Here's the drawing with two shaded views (mm, measured from the low corner). I have some questions. Round coordinates to 2 decimals unless told otherwise and drop trailing zeros.
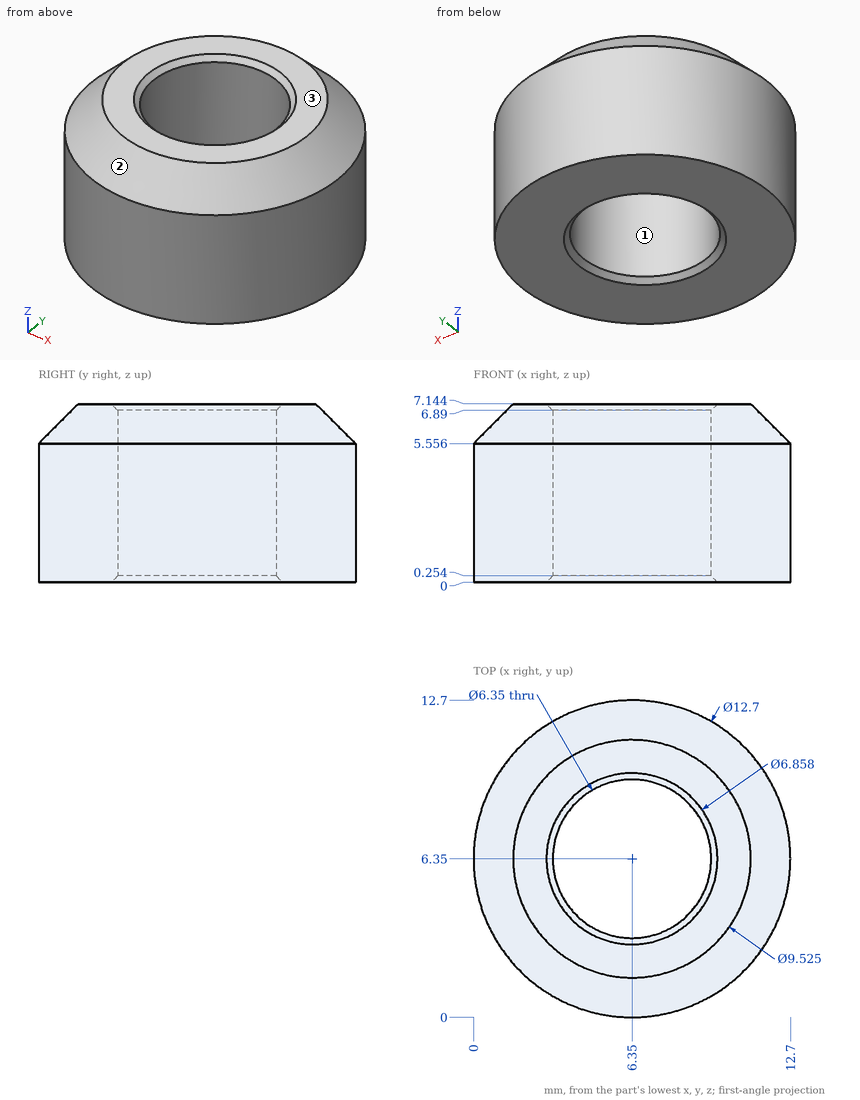
Item 1: Will these pins go through, and if not, where does the flat tip stop? pin 1 (5.5 mm diameter, centred on x = 6.35, y = 6.35, fed in from -Z); pin 2 (3 mm diameter, centred on x = 4, z = 6.5, fed in from -Y); pin 3 (2 mm diameter, centred on x = 3.5, z = 4, fed in from -Y) (1 decimal); pin 4 (2 mm diameter, centred on x = 10.5, z = 3, fed in from -Y).
Results list:
pin 1: passes through
pin 2: stops at y = 0.11
pin 3: stops at y = 0.3
pin 4: stops at y = 0.84
Item 2: If I drill on line 1 along Y through (x, z) = (6.35, 3.5) (1 decimal); line 2 along Y through (x, z) = (7.75, 0.75); line 3 along X through (y, z) = (8.75, 2.75), over which ranges is the centre line in solid material (lowest first)?
Results list:
line 1: y = 0 to 3.2, 9.5 to 12.7
line 2: y = 0.16 to 3.5, 9.2 to 12.54
line 3: x = 0.47 to 4.27, 8.43 to 12.23
Item 3: We'd pull the mould along X, two halves only. Please class the marked faces 1, 2 and 3: released by +X, released by -X, zero draft, split by the parting line, or undercut.
Results list:
face 1: undercut
face 2: split by the parting line
face 3: zero draft
